from build123d import *

# Parameters (mm, degrees)
SKETCH1_W           = 125
SKETCH1_H           = 155
SKETCH1_R           = 7.5
SKETCH1_W_2         = 15
SKETCH1_H_2         = 3
BOSS_EXTRUDE1_DEPTH = 3


with BuildPart() as part:
    # Sketch1 → Boss-Extrude1 (new body)
    with BuildSketch(Plane.XY):
        Rectangle(SKETCH1_W, SKETCH1_H)
        with Locations((0, -16)):
            Circle(SKETCH1_R, mode=Mode.SUBTRACT)
        with Locations((15, 73)):
            Rectangle(SKETCH1_W_2, SKETCH1_H_2, mode=Mode.SUBTRACT)
        with Locations((-40, 73)):
            Rectangle(SKETCH1_W_2, SKETCH1_H_2, mode=Mode.SUBTRACT)
        with Locations((-15, 73)):
            Rectangle(SKETCH1_W_2, SKETCH1_H_2, mode=Mode.SUBTRACT)
        with Locations((40, 73)):
            Rectangle(SKETCH1_W_2, SKETCH1_H_2, mode=Mode.SUBTRACT)
        with Locations((40, -73)):
            Rectangle(SKETCH1_W_2, SKETCH1_H_2, mode=Mode.SUBTRACT)
        with Locations((15, -73)):
            Rectangle(SKETCH1_W_2, SKETCH1_H_2, mode=Mode.SUBTRACT)
        with Locations((-15, -73)):
            Rectangle(SKETCH1_W_2, SKETCH1_H_2, mode=Mode.SUBTRACT)
        with Locations((-40, -73)):
            Rectangle(SKETCH1_W_2, SKETCH1_H_2, mode=Mode.SUBTRACT)
        with Locations((15, 41)):
            Rectangle(SKETCH1_W_2, SKETCH1_H_2, mode=Mode.SUBTRACT)
        with Locations((-15, 41)):
            Rectangle(SKETCH1_W_2, SKETCH1_H_2, mode=Mode.SUBTRACT)
        with BuildLine():
            Line((39.5, -10), (39.5, 9.186291501))
            ThreePointArc((39.5, 9.186291501), (37.648050297, 11.957930099), (34.378679656, 11.307611845))
            Line((34.378679656, 11.307611845), (16.655175669, -6.415892143))
            ThreePointArc((16.655175669, -6.415892143), (16.374485428, -6.967252196), (16.471908992, -7.578229748))
            ThreePointArc((16.471908992, -7.578229748), (17.443347183, -9.83723771), (18.106599572, -12.205128205))
            ThreePointArc((18.106599572, -12.205128205), (18.454909512, -12.776250026), (19.085334684, -13))
            Line((19.085334684, -13), (36.5, -13))
            ThreePointArc((36.5, -13), (38.621320344, -12.121320344), (39.5, -10))
        make_face(mode=Mode.SUBTRACT)
        with BuildLine():
            Line((3, -35.085334684), (3, -52.5))
            ThreePointArc((3, -52.5), (3.878679656, -54.621320344), (6, -55.5))
            Line((6, -55.5), (25.186291501, -55.5))
            ThreePointArc((25.186291501, -55.5), (27.957930099, -53.648050297), (27.307611845, -50.378679656))
            Line((27.307611845, -50.378679656), (9.584107857, -32.655175669))
            ThreePointArc((9.584107857, -32.655175669), (9.032747804, -32.374485428), (8.421770252, -32.471908992))
            ThreePointArc((8.421770252, -32.471908992), (6.16276229, -33.443347183), (3.794871795, -34.106599572))
            ThreePointArc((3.794871795, -34.106599572), (3.223749974, -34.454909512), (3, -35.085334684))
        make_face(mode=Mode.SUBTRACT)
        with BuildLine():
            Line((16.655175669, -25.584107857), (34.378679656, -43.307611845))
            ThreePointArc((34.378679656, -43.307611845), (37.648050297, -43.957930099), (39.5, -41.186291501))
            Line((39.5, -41.186291501), (39.5, -22))
            ThreePointArc((39.5, -22), (38.621320344, -19.878679656), (36.5, -19))
            Line((36.5, -19), (19.085334684, -19))
            ThreePointArc((19.085334684, -19), (18.454909512, -19.223749974), (18.106599572, -19.794871795))
            ThreePointArc((18.106599572, -19.794871795), (17.443347183, -22.16276229), (16.471908992, -24.421770252))
            ThreePointArc((16.471908992, -24.421770252), (16.374485428, -25.032747804), (16.655175669, -25.584107857))
        make_face(mode=Mode.SUBTRACT)
        with BuildLine():
            Line((6, 23.5), (25.186291501, 23.5))
            ThreePointArc((25.186291501, 23.5), (27.957930099, 21.648050297), (27.307611845, 18.378679656))
            Line((27.307611845, 18.378679656), (9.584107857, 0.655175669))
            ThreePointArc((9.584107857, 0.655175669), (9.032747804, 0.374485428), (8.421770252, 0.471908992))
            ThreePointArc((8.421770252, 0.471908992), (6.16276229, 1.443347183), (3.794871795, 2.106599572))
            ThreePointArc((3.794871795, 2.106599572), (3.223749974, 2.454909512), (3, 3.085334684))
            Line((3, 3.085334684), (3, 20.5))
            ThreePointArc((3, 20.5), (3.878679656, 22.621320344), (6, 23.5))
        make_face(mode=Mode.SUBTRACT)
        with BuildLine():
            Line((-3, 3.085334684), (-3, 20.5))
            ThreePointArc((-3, 20.5), (-3.878679656, 22.621320344), (-6, 23.5))
            Line((-6, 23.5), (-25.186291501, 23.5))
            ThreePointArc((-25.186291501, 23.5), (-27.957930099, 21.648050297), (-27.307611845, 18.378679656))
            Line((-27.307611845, 18.378679656), (-9.584107857, 0.655175669))
            ThreePointArc((-9.584107857, 0.655175669), (-9.032747804, 0.374485428), (-8.421770252, 0.471908992))
            ThreePointArc((-8.421770252, 0.471908992), (-6.16276229, 1.443347183), (-3.794871795, 2.106599572))
            ThreePointArc((-3.794871795, 2.106599572), (-3.223749974, 2.454909512), (-3, 3.085334684))
        make_face(mode=Mode.SUBTRACT)
        with BuildLine():
            Line((-39.5, -10), (-39.5, 9.186291501))
            ThreePointArc((-39.5, 9.186291501), (-37.648050297, 11.957930099), (-34.378679656, 11.307611845))
            Line((-34.378679656, 11.307611845), (-16.655175669, -6.415892143))
            ThreePointArc((-16.655175669, -6.415892143), (-16.374485428, -6.967252196), (-16.471908992, -7.578229748))
            ThreePointArc((-16.471908992, -7.578229748), (-17.443347183, -9.83723771), (-18.106599572, -12.205128205))
            ThreePointArc((-18.106599572, -12.205128205), (-18.454909512, -12.776250026), (-19.085334684, -13))
            Line((-19.085334684, -13), (-36.5, -13))
            ThreePointArc((-36.5, -13), (-38.621320344, -12.121320344), (-39.5, -10))
        make_face(mode=Mode.SUBTRACT)
        with BuildLine():
            Line((-19.085334684, -19), (-36.5, -19))
            ThreePointArc((-36.5, -19), (-38.621320344, -19.878679656), (-39.5, -22))
            Line((-39.5, -22), (-39.5, -41.186291501))
            ThreePointArc((-39.5, -41.186291501), (-37.648050297, -43.957930099), (-34.378679656, -43.307611845))
            Line((-34.378679656, -43.307611845), (-16.655175669, -25.584107857))
            ThreePointArc((-16.655175669, -25.584107857), (-16.374485428, -25.032747804), (-16.471908992, -24.421770252))
            ThreePointArc((-16.471908992, -24.421770252), (-17.443347183, -22.16276229), (-18.106599572, -19.794871795))
            ThreePointArc((-18.106599572, -19.794871795), (-18.454909512, -19.223749974), (-19.085334684, -19))
        make_face(mode=Mode.SUBTRACT)
        with BuildLine():
            Line((-3, -35.085334684), (-3, -52.5))
            ThreePointArc((-3, -52.5), (-3.878679656, -54.621320344), (-6, -55.5))
            Line((-6, -55.5), (-25.186291501, -55.5))
            ThreePointArc((-25.186291501, -55.5), (-27.957930099, -53.648050297), (-27.307611845, -50.378679656))
            Line((-27.307611845, -50.378679656), (-9.584107857, -32.655175669))
            ThreePointArc((-9.584107857, -32.655175669), (-9.032747804, -32.374485428), (-8.421770252, -32.471908992))
            ThreePointArc((-8.421770252, -32.471908992), (-6.16276229, -33.443347183), (-3.794871795, -34.106599572))
            ThreePointArc((-3.794871795, -34.106599572), (-3.223749974, -34.454909512), (-3, -35.085334684))
        make_face(mode=Mode.SUBTRACT)
        with BuildLine():
            Line((12.657211383, -0.372940136), (38.658474042, 25.628322523))
            ThreePointArc((38.658474042, 25.628322523), (41.628322523, 25.628322523), (41.628322523, 22.658474042))
            Line((41.628322523, 22.658474042), (15.627059864, -3.342788617))
            ThreePointArc((15.627059864, -3.342788617), (12.657211383, -3.342788617), (12.657211383, -0.372940136))
        make_face(mode=Mode.SUBTRACT)
        with BuildLine():
            Line((12.657211383, -31.627059864), (38.658474042, -57.628322523))
            ThreePointArc((38.658474042, -57.628322523), (41.628322523, -57.628322523), (41.628322523, -54.658474042))
            Line((41.628322523, -54.658474042), (15.627059864, -28.657211383))
            ThreePointArc((15.627059864, -28.657211383), (12.657211383, -28.657211383), (12.657211383, -31.627059864))
        make_face(mode=Mode.SUBTRACT)
        with BuildLine():
            Line((-12.657211383, -31.627059864), (-38.658474042, -57.628322523))
            ThreePointArc((-38.658474042, -57.628322523), (-41.628322523, -57.628322523), (-41.628322523, -54.658474042))
            Line((-41.628322523, -54.658474042), (-15.627059864, -28.657211383))
            ThreePointArc((-15.627059864, -28.657211383), (-12.657211383, -28.657211383), (-12.657211383, -31.627059864))
        make_face(mode=Mode.SUBTRACT)
        with BuildLine():
            Line((-12.657211383, -0.372940136), (-38.658474042, 25.628322523))
            ThreePointArc((-38.658474042, 25.628322523), (-41.628322523, 25.628322523), (-41.628322523, 22.658474042))
            Line((-41.628322523, 22.658474042), (-15.627059864, -3.342788617))
            ThreePointArc((-15.627059864, -3.342788617), (-12.657211383, -3.342788617), (-12.657211383, -0.372940136))
        make_face(mode=Mode.SUBTRACT)
        with Locations((40, 41)):
            Rectangle(SKETCH1_W_2, SKETCH1_H_2, mode=Mode.SUBTRACT)
        with Locations((-40, 43.5)):
            Rectangle(SKETCH1_W_2, SKETCH1_H_2, mode=Mode.SUBTRACT)
    extrude(amount=BOSS_EXTRUDE1_DEPTH)


solid = part.part
Part model, mm, in its own coordinate system. Coordinates: 2 decimals unless noted, no trailing zeros. Loops run counter-clockwise (first coordinate to the right, second up) from the corner with the lowest first, then second, coordinate; pieces in that order, holes last. Notation, with made-up numbers: (75.5, 78.25) -> (117.5, 78.25) arc R27 ccw to (117.5, 97.25) -> close; hole circle Ø2 at (77, 63). An arc over 180 degrees is marked (long way). Use a Markdown table: item, result. Add a question column.
Item 1: Pull direction Y, two halves, no side cores. Call faces 1 (the flat face through (-1, 77.5, 1)), 2 (the flat face through (-32.5, 43, 1)): +Y half, -Y half, draft (parallel to the pull), parting line (faces both ways), or undercut.
Item 2: Band-saw the part on B-B on x = 0. Write the cut outline in (y, z), plus the area to 3 significant figures.
Item 3: Probe probe 1 along Y at (x, z) = (0, 1.95); probe 2 along X at (y, z) = (16, 2); probe 3 along Y at (x, z) = (31.5, 1.95). List the from-to ranges inside material, lowest first.
Item 4: Flat gauge pin, fed straight in: P1, Ø6, axis at x = 38, y = -44.5, coming from the -Z side. Where does the tip first touch, or does it go through?
Item 5: Band-saw the part on C-C on z = 1.85. Give the number of separate pieces and of enclosed holes in the cut face, plus the area to 3 significant figures.
Item 6: Band-saw the part on A-A on y = -16. Write the cut outline in (x, z).
Geometry says:
| question | item | result |
|---|---|---|
| 1 | face 1 | +Y half |
| 1 | face 2 | undercut |
| 2 | outline | (-77.5, 0) -> (-23.5, 0) -> (-23.5, 3) -> (-77.5, 3) -> close; (-8.5, 0) -> (77.5, 0) -> (77.5, 3) -> (-8.5, 3) -> close |
| 2 | area | 420 mm² |
| 3 | probe 1 | -77.5 to -23.5, -8.5 to 77.5 |
| 3 | probe 2 | -62.5 to -34.97, -29.03 to -24.93, -3 to 3, 24.93 to 29.03, 34.97 to 62.5 |
| 3 | probe 3 | -77.5 to -50.47, -44.53 to -40.43, -19 to -13, 8.43 to 12.53, 18.47 to 77.5 |
| 4 | P1 | z = 0 |
| 5 | separate pieces | 1 |
| 5 | enclosed holes | 25 |
| 5 | area | 14,800 mm² |
| 6 | outline | (-62.5, 0) -> (-7.5, 0) -> (-7.5, 3) -> (-62.5, 3) -> close; (7.5, 0) -> (62.5, 0) -> (62.5, 3) -> (7.5, 3) -> close |
